Can you work these out from the model? Positions are in its coordinate system, mm. Face numbers are marked on the shaded views. A direction names the side the tool comes from. Give positions to 0.01 mm unless a question says otherwise; leave off trailing zeros. Loops run counter-clockwise (first coordinate to the right, second up) from the corner with the lowest first, then second, coordinate; pieces in that order, holes last. Notation, with made-up numbers: (37, 33) -> (80, 33) arc R25 ccw to (80, 70) -> close; hole circle Ø4 at (49.5, 69). An arc over 180 degrees is marked (long way). Use CSV: the item, a comma, the result in double quotes.
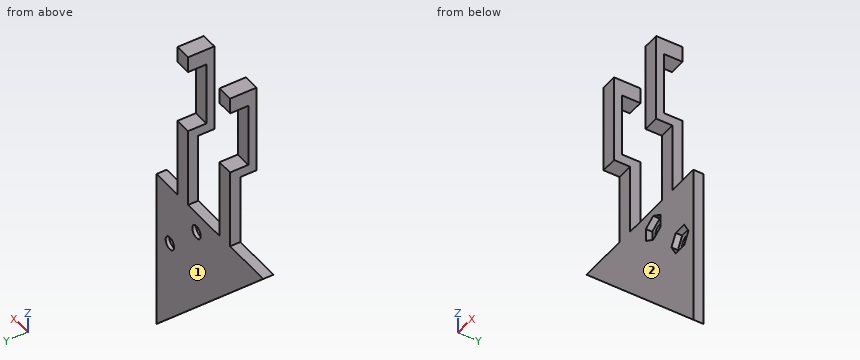
from build123d import *

# Parameters (mm, degrees)
BOSS_EXTRUDE1_DEPTH     = 3.175
SKETCH2_R               = 2
CUT_EXTRUDE1_DEPTH      = 72.912172996
CUT_EXTRUDE2_START      = -3.175
CUT_EXTRUDE2_DEPTH      = 2
BOSS_EXTRUDE2_START     = 10
BOSS_EXTRUDE2_DEPTH     = 5
BOSS_EXTRUDE3_START     = 30
BOSS_EXTRUDE3_DEPTH     = 5
CUT_EXTRUDE3_DEPTH      = 73.015831593
CUT_EXTRUDE3_DEPTH_BACK = 73.015831593
SKETCH6_W               = 50.943951029
SKETCH6_H               = 108.352089197


with BuildPart() as part:
    # Sketch1 → Boss-Extrude1 (new body)
    with BuildSketch(Plane(origin=(0, 0, 0), x_dir=(1, 0, 0), z_dir=(0, 1, 0))):
        Polygon((0, 0), (50.8, 0), (0, 50.8), align=None)
    extrude(amount=BOSS_EXTRUDE1_DEPTH)

    # Sketch2 → Cut-Extrude1 (cut, through all)
    with BuildSketch(Plane(origin=(0, 3.175, 0), x_dir=(1, 0, 0), z_dir=(0, 1, 0))):
        with Locations(Location((19.05, 6.35, 0), (0, 0, 270))):
            Circle(SKETCH2_R)
        with Locations(Location((6.35, 19.05, 0), (0, 0, 90))):
            Circle(SKETCH2_R)
    extrude(amount=-CUT_EXTRUDE1_DEPTH, mode=Mode.SUBTRACT)

    # Sketch3 → Cut-Extrude2 (cut)
    with BuildSketch(Plane(origin=(0, 3.175, 0), x_dir=(1, 0, 0), z_dir=(0, 1, 0)).offset(CUT_EXTRUDE2_START)):
        Polygon((8.370723055, 15.550005), (10.391446111, 19.05), (8.370723055, 22.549995), (4.329276945, 22.549995), (2.308553889, 19.05), (4.329276945, 15.550005), align=None)
        Polygon((22.549995, 4.329276945), (19.05, 2.308553889), (15.550005, 4.329276945), (15.550005, 8.370723055), (19.05, 10.391446111), (22.549995, 8.370723055), align=None)
    extrude(amount=CUT_EXTRUDE2_DEPTH, mode=Mode.SUBTRACT)

    # Sketch5 → Boss-Extrude2 (add)
    with BuildSketch(Plane(origin=(0, 0, 0), x_dir=(0, 0, -1), z_dir=(1, 0, 0)).offset(BOSS_EXTRUDE2_START)):
        Polygon((0, 0), (0, 3.175), (-25, 3.175), (-25, -2.5), (-45, -2.5), (-45, 3.175), (-50, 3.175), (-50, -5), (-22, -5), (-22, 0), align=None)
    extrude(amount=BOSS_EXTRUDE2_DEPTH)

    # Sketch5<3> → Boss-Extrude3 (add)
    with BuildSketch(Plane(origin=(0, 0, 0), x_dir=(0, 0, -1), z_dir=(1, 0, 0)).offset(BOSS_EXTRUDE3_START)):
        Polygon((0, 0), (0, 3.175), (-25, 3.175), (-25, -2.5), (-45, -2.5), (-45, 3.175), (-50, 3.175), (-50, -5), (-22, -5), (-22, 0), align=None)
    extrude(amount=BOSS_EXTRUDE3_DEPTH)

    # Mirror1: part across plane


with BuildPart() as part_1:
    add(part.part)
    add(part.part.mirror(Plane(origin=(0, 0, 0), x_dir=(0, 0, 1), z_dir=(1, 0, 0))))

    # Sketch6 → Cut-Extrude3 (cut, two sides: drawn at the far end of the back side and taken through both)
    with BuildSketch(Plane(origin=(0, 0, 0), x_dir=(1, 0, 0), z_dir=(0, 1, 0)).offset(-CUT_EXTRUDE3_DEPTH_BACK)):
        with Locations((25.471975515, -0.138682261)):
            Rectangle(SKETCH6_W, SKETCH6_H)
    extrude(amount=CUT_EXTRUDE3_DEPTH + CUT_EXTRUDE3_DEPTH_BACK, mode=Mode.SUBTRACT)


solid = part_1.part
(1) If I drill on L1, parallel to X at y = 0.75, z = 16; L2, parallel to Z at x = -13, y = -0.25; L3, parallel to Y at x = -39.5, z = -1 (3 decimals), over which ranges is the centre line in solid material (lowest first)? Write a range as from..to.
Answer sheet:
L1,"x = -35..-30, -15..-10"
L2,"z = 22..25, 45..50"
L3,"y = 0..3.175"
(2) If we section it at B-B, the plane y = -3.5: Write out the boundary of the cut face in (x, z), then the cut area to 3 significant figures.
Answer sheet:
outline,"(-35, 22) -> (-30, 22) -> (-30, 50) -> (-35, 50) -> close; (-15, 22) -> (-10, 22) -> (-10, 50) -> (-15, 50) -> close"
area,"280 mm2"
(3) If we section it at D-D, the plane z = 7.5: Write out the boundary of the cut face in (x, y) (3 decimals), then the cut area to 4 significant figures.
Answer sheet:
outline,"(-35, 0) -> (-30, 0) -> (-30, 3.175) -> (-35, 3.175) -> close; (-15, 0) -> (-10, 0) -> (-10, 3.175) -> (-15, 3.175) -> close"
area,"31.75 mm2"
(4) If we section it at A-A, the plane z = -6.35: Write out the boundary of the cut face in (x, y) (3 decimals), then the cut area to 3 significant figures.
Answer sheet:
outline,"(-44.45, 0) -> (-22.55, 0) -> (-22.55, 2) -> (-21.05, 2) -> (-21.05, 3.175) -> (-44.45, 3.175) -> close; (-17.05, 2) -> (-15.55, 2) -> (-15.55, 0) -> (0, 0) -> (0, 3.175) -> (-17.05, 3.175) -> close"
area,"122 mm2"
(5) Will these pins go through, and if not, where does the flat tip stop? pin 1 Ø1.5 at (x, y) = (-32.5, -3) entering from -Z; pin 2 Ø1 at (x, y) = (-5, 1) entering from +Z; pin 3 Ø6 at (x, z) = (-16.5, -21.5) entering from -Y; pin 4 Ø2.5 at (x, z) = (-6.35, -19.05) entering from -Y.
Answer sheet:
pin 1,"stops at z = 22"
pin 2,"stops at z = 0"
pin 3,"stops at y = 0"
pin 4,"passes through"
(6) Which directions (+Z, -Z, +X, -X, +Y, -Y) give clear straight access to the entire face, cutting with the end or side of a thin tool? Please do the marked faces 1 and 2.
Answer sheet:
face 1,"+Z, -Z, +X, -X, +Y"
face 2,"-Z, +X, -X, -Y"
(7) If we section it at C-C, the plane x = -6.35: Write out the boundary of the cut face in (y, z) (3 decimals), then the cut area to 3 significant figures.
Answer sheet:
outline,"(0, -44.45) -> (3.175, -44.45) -> (3.175, -21.05) -> (2, -21.05) -> (2, -22.55) -> (0, -22.55) -> close; (0, -15.55) -> (2, -15.55) -> (2, -17.05) -> (3.175, -17.05) -> (3.175, 0) -> (0, 0) -> close"
area,"122 mm2"
